Build history of the part. All positions in model axes, mm. A direction names the side the tool comes from. Give positions to 0.01 mm unless a question says otherwise; leave off trailing zeros. Order: outer loops, then holes, each group sorted by start corner. A loop starts at its lowest first (then second) coordinate and runs counter-clockwise, first axis right, second up. Notation, with made-up numbers: M -40,69.25 L -30,69.25 A25 ccw -30,104.25 Z; hole C 13.5,62.25 d9. An arc over 180 degrees is marked long. Use CSV: the item, a comma, the result in double quotes. Start each with the question number.
Item 1: Two-plate mould, pull along Y, no slides. Class faces 4 (the flat face through (31, 0, 67)), 5 (the cylindrical face through (9.805, 21.514, 59.487)), 6 (the flat face through (34, 37, 21)), 7 (the flat face through (10, 20.5, 56)): pulls with the +Y half, pulls with the -Y half, needs draft (parallel to the pull), parting line crosses it, or undercut.
Item 2: Which spindle directions (+Z, -Z, +X, -X, +Y, -Y) get a long thin tool onto all of the face, cutting with end or side? Do faces 1 (the flat face through (66, 15, 34)), 2 (the cylindrical face through (57.43, 5.45, 1.01)), 3 (the flat face through (19, 37, 34)). Say none if no direction does.
Item 3: Band-saw the part on D-D on z = 11. Write the cut outline in (x, y), plus the area to 3 significant figures.
Item 4: Band-saw the part on C-C on z = 34. Write the cut outline in (x, y).
Item 5: Band-saw the part on A-A on x = 56. Write the cut outline in (y, z).
Item 6: Wall check: line 1 along X through (y, z) = (36, 34); line 2 along Z through (x, y) = (62.5, 5.5); line 3 along X through (y, z) = (31.2, 34). Give the ranges that are in metal, low to high.
Item 7: Band-saw the part on B-B on y = 28. Write the cut outline in (x, z).
Item 8: Pin check, flat tips, straight feed: P1, Ø5.5, axis at x = 9, z = 57.5, coming from the -Y side; P2, Ø4, axis at x = 33.5, z = 39, coming from the +Y side; P3, Ø1.8, axis at x = 56, y = 5, coming from the -Z side. Stop position of each tip, or through.
from build123d import *

# Parameters (mm, degrees)
SKETCH2_W           = 68
SKETCH2_H           = 68
BOSS_EXTRUDE1_DEPTH = 38
SKETCH3_W           = 64
SKETCH3_H           = 64
CUT_EXTRUDE1_DEPTH  = 30
SKETCH5_W           = 30
SKETCH5_H           = 30
SKETCH5_W_2         = 26
SKETCH5_H_2         = 26
CUT_EXTRUDE2_DEPTH  = 3
SKETCH6_R           = 6.05
CUT_EXTRUDE3_DEPTH  = 39
SKETCH7_R           = 10.5
CUT_EXTRUDE4_DEPTH  = 5
SKETCH8_R           = 1.5
CUT_EXTRUDE5_DEPTH  = 3
SKETCH9_R           = 2.5
BOSS_EXTRUDE2_DEPTH = 7.5
SKETCH10_R          = 1.5
BOSS_EXTRUDE3_DEPTH = 2
SKETCH11_R          = 2.5
BOSS_EXTRUDE4_DEPTH = 2


with BuildPart() as part:
    # Sketch2 → Boss-Extrude1 (new body)
    with BuildSketch(Plane(origin=(0, 0, 0), x_dir=(1, 0, 0), z_dir=(0, 1, 0))):
        with Locations((34, -34)):
            Rectangle(SKETCH2_W, SKETCH2_H)
    extrude(amount=BOSS_EXTRUDE1_DEPTH)

    # Sketch3 → Cut-Extrude1 (cut)
    with BuildSketch(Plane.XZ):
        with Locations((34, 34)):
            Rectangle(SKETCH3_W, SKETCH3_H)
    extrude(amount=-CUT_EXTRUDE1_DEPTH, mode=Mode.SUBTRACT)

    # Sketch5 → Cut-Extrude2 (cut)
    with BuildSketch(Plane(origin=(0, 38, 0), x_dir=(1, 0, 0), z_dir=(0, 1, 0))):
        with Locations((34, -34)):
            Rectangle(SKETCH5_W, SKETCH5_H)
        with Locations((34, -34)):
            Rectangle(SKETCH5_W_2, SKETCH5_H_2, mode=Mode.SUBTRACT)
    extrude(amount=-CUT_EXTRUDE2_DEPTH, mode=Mode.SUBTRACT)

    # Sketch6 → Cut-Extrude3 (cut, through all)
    with BuildSketch(Plane(origin=(0, 38, 0), x_dir=(1, 0, 0), z_dir=(0, 1, 0))):
        with Locations((34, -34)):
            Circle(SKETCH6_R)
    extrude(amount=-CUT_EXTRUDE3_DEPTH, mode=Mode.SUBTRACT)

    # Sketch7 → Cut-Extrude4 (cut)
    with BuildSketch(Plane(origin=(0, 38, 0), x_dir=(1, 0, 0), z_dir=(0, 1, 0))):
        with Locations((34, -34)):
            Circle(SKETCH7_R)
    extrude(amount=-CUT_EXTRUDE4_DEPTH, mode=Mode.SUBTRACT)

    # Sketch8 → Cut-Extrude5 (cut, through all)
    with BuildSketch(Plane.XY.offset(2)):
        with Locations((56, 5)):
            Circle(SKETCH8_R)
    extrude(amount=-CUT_EXTRUDE5_DEPTH, mode=Mode.SUBTRACT)

    # Sketch9 → Boss-Extrude2 (add)
    with BuildSketch(Plane.XZ.offset(-30)):
        with Locations((10, 58)):
            Circle(SKETCH9_R)
    extrude(amount=BOSS_EXTRUDE2_DEPTH)

    # Sketch10 → Boss-Extrude3 (add)
    with BuildSketch(Plane.XZ.offset(-22.5)):
        with Locations((10, 58)):
            Circle(SKETCH10_R)
    extrude(amount=BOSS_EXTRUDE3_DEPTH)

    # Sketch11 → Boss-Extrude4 (add)
    with BuildSketch(Plane.XZ.offset(-20.5)):
        with Locations((10, 58)):
            Circle(SKETCH11_R)
    extrude(amount=BOSS_EXTRUDE4_DEPTH)


solid = part.part
Model answer:
1,face 4,"pulls with the -Y half"
1,face 5,"undercut"
1,face 6,"needs draft"
1,face 7,"undercut"
2,face 1,"-Y"
2,face 2,"-Z"
2,face 3,"+Y"
3,outline,"M 0,0 L 2,0 L 2,30 L 66,30 L 66,0 L 68,0 L 68,38 L 0,38 Z"
3,area,"664 mm^2"
4,outline,"M 0,0 L 2,0 L 2,30 L 27.95,30 L 27.95,33 L 23.5,33 L 23.5,38 L 21,38 L 21,35 L 19,35 L 19,38 L 0,38 Z; M 40.05,30 L 66,30 L 66,0 L 68,0 L 68,38 L 49,38 L 49,35 L 47,35 L 47,38 L 44.5,38 L 44.5,33 L 40.05,33 Z"
5,outline,"M 0,0 L 3.5,0 L 3.5,2 L 0,2 Z; M 0,66 L 30,66 L 30,2 L 6.5,2 L 6.5,0 L 38,0 L 38,68 L 0,68 Z"
6,line 1,"x = 0 to 19, 21 to 23.5, 44.5 to 47, 49 to 68"
6,line 2,"z = 0 to 2, 66 to 68"
6,line 3,"x = 0 to 27.95, 40.05 to 68"
7,outline,"M 0,0 L 68,0 L 68,68 L 0,68 Z; C 10,58 d5; hole M 2,2 L 66,2 L 66,66 L 2,66 Z"
8,P1,"stops at y = 18.5"
8,P2,"stops at y = 33"
8,P3,"stops at z = 66"
